```python
from build123d import *

# Parameters (mm, degrees)
F0_R     = 18.9865
F1_DEPTH = 38.1
F2_SIZE  = 0.79375
F4_DEPTH = 4.572
F5_R     = 18.19275
F6_DEPTH = 101.6
F7_R     = 6.35
F8_DEPTH = 38.1


with BuildPart() as f1:
    # F0 (on Top) → F1 (new body, symmetric)
    with BuildSketch(Plane.XY):
        Circle(F0_R)
    extrude(amount=F1_DEPTH, both=True)

    # F2
    f2_edges = [f1.edges().sort_by_distance(p)[0] for p in [
        (-18.9865, 0, 38.1),
        (-18.9865, 0, -38.1),
    ]]
    chamfer(f2_edges, length=F2_SIZE)

    # F3 (on Right) → F4 (cut, symmetric)
    with BuildSketch(Plane.YZ):
        with BuildLine():
            Line((19.05, 38.1), (13.97, 38.1))
            Line((13.97, 38.1), (13.97, -12.7))
            ThreePointArc((13.97, -12.7), (15.4013111503, -16.7160926284), (19.05, -18.9217039467))
            Line((19.05, -18.9217039467), (19.05, 38.1))
        make_face()
    extrude(amount=F4_DEPTH, both=True, mode=Mode.SUBTRACT)

    # F5 (on face) → F6 (join)
    with BuildSketch(Plane(origin=(0, 0, -38.1), x_dir=(1, 0, 0), z_dir=(0, 0, -1))):
        Circle(F5_R)
    extrude(amount=F6_DEPTH)

    # F7 (on Front) → F8 (cut, symmetric)
    with BuildSketch(Plane.XZ):
        with Locations((0, -127)):
            Circle(F7_R)
    extrude(amount=F8_DEPTH, both=True, mode=Mode.SUBTRACT)


solid = f1.part
```
The model under review builds one solid part; all positions refer to its coordinate system, in mm. A direction names the side the tool comes from. Round coordinates to 2 decimals unless told otherwise and drop trailing zeros. Loops run counter-clockwise (first coordinate to the right, second up) from the corner with the lowest first, then second, coordinate; pieces in that order, holes last.
1) Consider section A-A on x = 0. State the section outline as (y, z) points, then the cut area to 3 significant figures.
Values follow:
outline: (-18.99, -37.31) - (-18.19, -38.1) - (-18.19, -120.65) - (18.19, -120.65) - (18.19, -38.1) - (18.99, -37.31) - (18.99, -18.91) arc R6.35 cw to (13.97, -12.7) - (13.97, 38.1) - (-18.19, 38.1) - (-18.99, 37.31) - close; (-18.19, -139.7) - (18.19, -139.7) - (18.19, -133.35) - (-18.19, -133.35) - close
area: 5,850 mm2
2) Clearance check with flat-ended pins moving along their axes: P1, Ø2, axis at x = 8.5, z = -11.5, coming from the -Y side; P2, Ø6, axis at x = -11.5, z = -62.5, coming from the +Y side; P3, Ø5, axis at x = 13.5, z = -25.5, coming from the +Y side; P4, Ø7.5, axis at x = 0, z = -127, coming from the -Y side. State where each tip first meets the part, or that it passes through.
Values follow:
P1: stops at y = -17.44
P2: stops at y = 16.08
P3: stops at y = 15.48
P4: passes through
3) Consider section C-C on z = -63. State the section outline as (x, y) points.
Values follow:
outline: circle Ø36.39 at (0, 0)
4) Consider section D-D on z = 27. State the section outline as (x, y) points.
Values follow:
outline: (-4.57, 13.97) - (-4.57, 18.43) arc R18.99 ccw (long way) to (4.57, 18.43) - (4.57, 13.97) - close
5) The part is to be moulded in two halves that separate along Z. For faces 4 (the face through (0, 13.97, 13)), 5 (the face through (3.414, -0.255, -121.646)), 6 (the face through (0, 0, -139.7)), say which applies: pulls with the +Z half, pulls with the -Z half, needs draft (parallel to the pull), parting line crosses it, or undercut.
Values follow:
face 4: needs draft
face 5: undercut
face 6: pulls with the -Z half
6) Consider section B-B on z = -127. State the section outline as (x, y) points, then the cut area to 3 significant figures.
Values follow:
outline: (-6.35, -17.05) - (-6.35, 17.05) arc R18.19 ccw to start; (6.35, -17.05) arc R18.19 ccw to (6.35, 17.05) - close
area: 587 mm2
7) Wall thickness on line 1 along Z through (x, y) = (0, -9); line 2 along X through (y, z) = (-6, -127); line 3 along X through (y, z) = (-3.5, -127): over which ranges is each line inside the solid? List them lowest first.
Values follow:
line 1: z = -139.7 to -133.35, -120.65 to 38.1
line 2: x = -17.17 to -6.35, 6.35 to 17.17
line 3: x = -17.85 to -6.35, 6.35 to 17.85
8) Tool access review of faces 1 (the face through (4.572, 16, 10)), 2 (the face through (-4.116, -18.535, 0.522)), 3 (the face through (16.805, 6.968, -88.189)): name each direction out of +Z, -Z, +X, -X, +Y, -Y from which nothing blocks a thin tool from reaching the whole face with its end or side.
Values follow:
face 1: +Z, +Y
face 2: +Z, -Z
face 3: -Z
